from build123d import *

# Parameters (mm, degrees)
SKETCH1_W                    = 106
SKETCH1_H                    = 50
BASE_FLANGE1_DEPTH           = 8
EDGE_FLANGE1_STRIP_W         = 48
EDGE_FLANGE1_STRIP_H         = 8
EDGE_FLANGE1_STRIP_CUT_DEPTH = 106
EDGE_FLANGE1_DEPTH           = 106
CHAMFER1_SIZE                = 43
CHAMFER1_SIZE2               = 30.108924143
MIRROR3_START                = 33.090682493
MIRROR3_OUTLINE_W            = 56
MIRROR3_OUTLINE_H            = 41
MIRROR3_DEPTH                = 24.663786763


# Read off the part's stored shape, not the designer's step: Mirror3
# Sheet-metal steps are written as plain solids
with BuildPart() as part:
    # Sketch1 → Base-Flange1 (new body)
    with BuildSketch(Plane(origin=(0, 0, 0), x_dir=(1, 0, 0), z_dir=(0, 1, 0))):
        Rectangle(SKETCH1_W, SKETCH1_H)
    extrude(amount=-BASE_FLANGE1_DEPTH)

    # Edge-Flange1 strip (across the edge) → Edge-Flange1 strip cut (cut)
    with BuildSketch(Plane(origin=(-53, 0, 25), x_dir=(0, 0, -1), z_dir=(1, 0, 0))):
        with Locations((-8, -4)):
            Rectangle(EDGE_FLANGE1_STRIP_W, EDGE_FLANGE1_STRIP_H)
    extrude(amount=EDGE_FLANGE1_STRIP_CUT_DEPTH, mode=Mode.SUBTRACT)

    # Edge-Flange1 section (across the edge) → Edge-Flange1 (add)
    with BuildSketch(Plane(origin=(-53, 0, 25), x_dir=(0, 0, -1), z_dir=(1, 0, 0))):
        with BuildLine():
            Line((0, 8), (0, 32))
            Line((0, 32), (8, 32))
            Line((8, 32), (8, 8))
            ThreePointArc((8, 8), (10.343145751, 2.343145751), (16, 0))
            Line((16, 0), (16, -8))
            ThreePointArc((16, -8), (4.686291501, -3.313708499), (0, 8))
        make_face()
    extrude(amount=EDGE_FLANGE1_DEPTH)

    # Chamfer1
    chamfer1_edges = [part.edges().sort_by_distance(p)[0] for p in [
        (-53, -4, -25),
    ]]
    chamfer1_side = [part.faces().sort_by_distance(p)[0] for p in [
        (-53, -0.640312424, -8),
    ]]
    chamfer(chamfer1_edges, length=CHAMFER1_SIZE, length2=CHAMFER1_SIZE2, reference=chamfer1_side[0])

    # Mirror3 outline → Mirror3 (cut)
    with BuildSketch(Plane(origin=(0, 0, 0), x_dir=(0.5735764363510512, 0, 0.8191520442889882), z_dir=(0.8191520442889882, 0, -0.5735764363510512)).offset(MIRROR3_START)):
        with Locations((19, -12.5)):
            Rectangle(MIRROR3_OUTLINE_W, MIRROR3_OUTLINE_H)
    extrude(amount=MIRROR3_DEPTH, mode=Mode.SUBTRACT)


solid = part.part
Check sheet for the modelled part. Datum: model origin and axes. Units: mm. A direction names the side the tool comes from. Coordinates: 2 decimals unless noted, no trailing zeros. Loops run counter-clockwise (first coordinate to the right, second up) from the corner with the lowest first, then second, coordinate; pieces in that order, holes last. Notation, with made-up numbers: (-15.75, 80) -> (38.25, 80) arc R19 ccw to (38.25, 110) -> close; hole circle Ø7 at (67.25, 27). An arc over 180 degrees is marked (long way). Answer in a Markdown table with one row per item.
1. Sectioned sample at C-C, the plane z = 0.5. Record the boundary of the cut face in (x, y).
Check values:
| item | result |
|---|---|
| outline | (-40.75, -8) -> (40.75, -8) -> (40.75, 0) -> (-40.75, 0) -> close |
2. Material ranges on line 1 along Z through (x, y) = (15, 28); line 2 along Y through (x, z) = (15, 0.5); line 3 along Y through (x, z) = (3, 18), recorded low to high. Write a range as [from, to].
Check values:
| item | result |
|---|---|
| line 1 | z = [17, 25] |
| line 2 | y = [-8, 0] |
| line 3 | y = [-5.23, 32] |
3. Sectioned sample at B-B, the plane y = 11.5. Record the boundary of the cut face in (x, z), then the cut area to 3 significant figures.
Check values:
| item | result |
|---|---|
| outline | (-53, 18) -> (-52.3, 17) -> (52.3, 17) -> (53, 18) -> (53, 25) -> (-53, 25) -> close |
| area | 847 mm2 |
4. Access from +Z, -Z, +X, -X, +Y, -Y to the whole of each face (thin tool, end or side, straight path). Record for faces 1 (the face through (-1, -8, -4)), 2 (the face through (-1, 0, -4)).
Check values:
| item | result |
|---|---|
| face 1 | +Z, -Z, +X, -X, -Y |
| face 2 | -Z, +X, -X, +Y |
5. Go/stop test with flat-tipped pins: pin 1 (1 mm diameter, centred on x = 15.5, y = 9.5, fed in from -Z); pin 2 (1 mm diameter, centred on x = -20.5, z = 15, fed in from -Y) (3 decimals); pin 3 (8 mm diameter, centred on x = -4.5, y = -1.5, fed in from +Z) (3 decimals). Record where each tip stops, or that it passes through.
Check values:
| item | result |
|---|---|
| pin 1 | stops at z = 17 |
| pin 2 | stops at y = -7.025 |
| pin 3 | stops at z = 24.025 |
6. Sectioned sample at D-D, the plane x = 13.5. Record the boundary of the cut face in (y, z), then the cut area to 3 significant figures.
Check values:
| item | result |
|---|---|
| outline | (-8, -25) -> (0, -25) -> (0, 9) arc R8 cw to (8, 17) -> (32, 17) -> (32, 25) -> (8, 25) arc R16 ccw to (-8, 9) -> close |
| area | 615 mm2 |
7. Sectioned sample at A-A, the plane x = -26. Record the boundary of the cut face in (y, z), then the cut area to 3 significant figures.
Check values:
| item | result |
|---|---|
| outline | (-8, -20.56) -> (0, -20.56) -> (0, 9) arc R8 cw to (8, 17) -> (32, 17) -> (32, 25) -> (8, 25) arc R16 ccw to (-8, 9) -> close |
| area | 579 mm2 |
